from build123d import *

# Parameters (mm, degrees)
EXTRUDE_1_DEPTH     = 20
SKETCH_2_R          = 1.5
CUT_EXTRUDE_1_DEPTH = 20
SKETCH_3_R          = 7.5
EXTRUDE_2_DEPTH     = 50
EXTRUDE_3_DEPTH     = 10
SKETCH_7_W          = 18
SKETCH_7_H          = 39
EXTRUDE_4_DEPTH     = 5
SKETCH_9_R          = 5
SKETCH_9_R_2        = 1.75
CUT_EXTRUDE_2_DEPTH = 15
SKETCH_12_R         = 4
CUT_EXTRUDE_3_DEPTH = 20
CUT_EXTRUDE_START   = -60.849857
SKETCH_13_W         = 10
SKETCH_13_H         = 24
CUT_EXTRUDE_4_DEPTH = 60.849857
SKETCH_14_R         = 1.75
CUT_EXTRUDE_5_DEPTH = 10


with BuildPart() as part:
    # 草图1 → 凸台-拉伸1 (new body)
    with BuildSketch(Plane.XY):
        Polygon((-18, 29.079835166), (-13.000041786, 24.079835166), (-13.000343311, -12.000164834), (-10.85, -12.000164834), (-8.85, -14.000164834), (11.15, -14.000164834), (13.15, -12.000164834), (19.15, -12.000164834), (21.15, -14.000164834), (21.15, -28.920164834), (-73.85, -28.920164834), (-73.85, 29.079835166), align=None)
    extrude(amount=EXTRUDE_1_DEPTH)

    # 草图2 → 切除-拉伸1 (cut)
    with BuildSketch(Plane.XY.offset(20)):
        with Locations((-15.5, 15.5)):
            Circle(SKETCH_2_R)
        with Locations((-15.5, -15.5)):
            Circle(SKETCH_2_R)
        with Locations((15.5, -15.5)):
            Circle(SKETCH_2_R)
    extrude(amount=-CUT_EXTRUDE_1_DEPTH, mode=Mode.SUBTRACT)

    # 草图3 → 凸台-拉伸2 (add)
    with BuildSketch(Plane.XZ.offset(28.920164834)):
        with BuildLine():
            Line((-43.15, 31), (-43.15, 20))
            Line((-43.15, 20), (-21.15, 20))
            Line((-21.15, 20), (-21.15, 31))
            ThreePointArc((-21.15, 31), (-32.15, 42), (-43.15, 31))
        make_face()
        with Locations((-32.15, 31)):
            Circle(SKETCH_3_R, mode=Mode.SUBTRACT)
    extrude(amount=-EXTRUDE_2_DEPTH)

    # 草图5 → 凸台-拉伸3 (add)
    with BuildSketch(Plane.XZ.offset(28.920164834)):
        with BuildLine():
            Line((-43.15, 42), (-32.15, 42))
            ThreePointArc((-32.15, 42), (-39.928174593, 38.778174593), (-43.15, 31))
            Line((-43.15, 31), (-43.15, 20))
            Line((-43.15, 20), (-65.15, 20))
            Line((-65.15, 20), (-65.15, 37))
            ThreePointArc((-65.15, 37), (-63.685533906, 40.535533906), (-60.15, 42))
            Line((-60.15, 42), (-43.15, 42))
        make_face()
    extrude(amount=-EXTRUDE_3_DEPTH)

    # 草图7 → 凸台-拉伸4 (add)
    with BuildSketch(Plane.XY.offset(20)):
        with Locations((-82.85, -9.420164834)):
            Rectangle(SKETCH_7_W, SKETCH_7_H)
    extrude(amount=-EXTRUDE_4_DEPTH)

    # 草图9 → 切除-拉伸2 (cut)
    with BuildSketch(Plane.XZ.offset(28.920164834)):
        with Locations((-54.15, 31)):
            Circle(SKETCH_9_R)
        with Locations((-59.806854249, 36.656854249)):
            Circle(SKETCH_9_R_2)
        with Locations((-48.493145751, 36.656854249)):
            Circle(SKETCH_9_R_2)
        with Locations((-48.493145751, 25.343145751)):
            Circle(SKETCH_9_R_2)
        with Locations((-59.806854249, 25.343145751)):
            Circle(SKETCH_9_R_2)
    extrude(amount=-CUT_EXTRUDE_2_DEPTH, mode=Mode.SUBTRACT)

    # 草图12 → 切除-拉伸3 (cut)
    with BuildSketch(Plane.ZY.offset(73.85)):
        with Locations((10, 22.579835166)):
            Circle(SKETCH_12_R)
        with Locations((10, -22.420164834)):
            Circle(SKETCH_12_R)
    extrude(amount=-CUT_EXTRUDE_3_DEPTH, mode=Mode.SUBTRACT)

    # 草图13 → 切除-拉伸4 (cut)
    with BuildSketch(Plane.ZY.offset(73.85).offset(CUT_EXTRUDE_START)):
        with Locations((10, 0)):
            Rectangle(SKETCH_13_W, SKETCH_13_H)
    extrude(amount=CUT_EXTRUDE_4_DEPTH, mode=Mode.SUBTRACT)

    # 草图14 → 切除-拉伸5 (cut)
    with BuildSketch(Plane.XY.offset(20)):
        with Locations((-88.6, -12.170164834)):
            Circle(SKETCH_14_R)
        with Locations((-88.6, 6.829835166)):
            Circle(SKETCH_14_R)
    extrude(amount=-CUT_EXTRUDE_5_DEPTH, mode=Mode.SUBTRACT)


solid = part.part
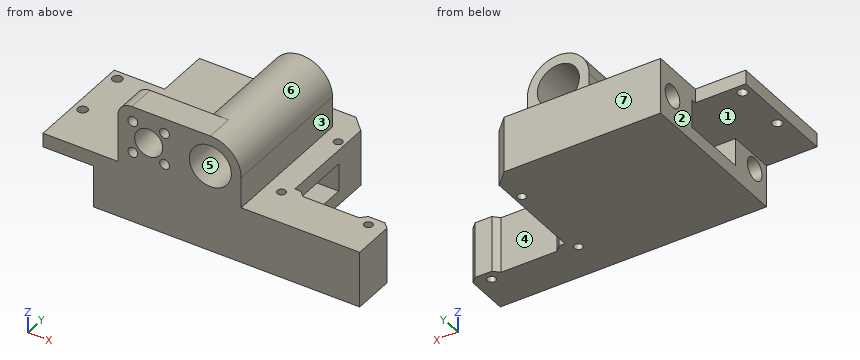
Part model, mm, in its own coordinate system. Face numbers are marked on the shaded views. A direction names the side the tool comes from. Coordinates: 2 decimals unless noted, no trailing zeros. Loops run counter-clockwise (first coordinate to the right, second up) from the corner with the lowest first, then second, coordinate; pieces in that order, holes last. Notation, with made-up numbers: (21.5, 71) -> (48.5, 71) arc R20 cw to (48.5, 78) -> close; hole circle Ø2 at (43, -16). An arc over 180 degrees is marked (long way). Use a Markdown table: item, result. Add a question column.
Item 1: Which spindle directions (+Z, -Z, +X, -X, +Y, -Y) get a long thin tool onto all of the face, cutting with end or side? Do the marked faces 1, 2, 3 and 4. Say none if no direction does.
Item 2: Band-saw the part on C-C on x = -88.6. Write the cut outline in (y, z).
Item 3: Probe probe 1 along Y at (x, z) = (-15.5, 4.75); probe 2 along Z at (x, y) = (-32.15, 0.5); probe 3 along Y at (x, z) = (-59, 10). List the from-to ranges inside material, lowest first.
Item 4: Band-saw the part on A-A on z = 10. Give the number of separate pieces and of enclosed holes in the cut face, plus the area to 3 significant figures.
Item 5: Band-saw the part on B-B on y = 15.5. Write the cut outline in (x, z), plus the area to 3 significant figures.
Item 6: Band-saw the part on D-D on z = 3. Write the cut outline in (x, y), plus the area to 3 significant figures.
Item 7: Flat gauge pins, fed straight in: P1, Ø17.5, axis at x = -29, z = 29.5, coming from the +Y side; P2, Ø3, axis at x = -76.5, y = 22.5, coming from the +Z side; P3, Ø3, axis at x = 15, z = 14, coming from the +Y side; P4, Ø9, axis at y = 22.5, z = 9.5, coming from the -X side. Where does each tip first touch, or does it go through?
Item 8: Pull direction X, two halves, no side cores. Call the marked faces 5, 6 and 7: +X half, -X half, draft (parallel to the pull), parting line (faces both ways), or undercut.
Geometry says:
| question | item | result |
|---|---|---|
| 1 | face 1 | -X |
| 1 | face 2 | -Z, -X, +Y |
| 1 | face 3 | +Z, +X, +Y, -Y |
| 1 | face 4 | +Z, -Z, +Y |
| 2 | outline | (-28.92, 15) -> (-13.92, 15) -> (-13.92, 20) -> (-28.92, 20) -> close; (-10.42, 15) -> (5.08, 15) -> (5.08, 20) -> (-10.42, 20) -> close; (8.58, 15) -> (10.08, 15) -> (10.08, 20) -> (8.58, 20) -> close |
| 3 | probe 1 | -28.92 to -17, -14 to 14, 17 to 26.58 |
| 3 | probe 2 | 0 to 5, 15 to 23.5, 38.5 to 42 |
| 3 | probe 3 | -28.92 to -26.42, -18.42 to -12, 12 to 18.58, 26.58 to 29.08 |
| 4 | separate pieces | 2 |
| 4 | enclosed holes | 3 |
| 4 | area | 2,250 mm² |
| 5 | outline | (-73.85, 0) -> (-17, 0) -> (-17, 20) -> (-21.15, 20) -> (-21.15, 31) arc R11 ccw to (-43.15, 31) -> (-43.15, 20) -> (-73.85, 20) -> close; (-14, 0) -> (-13, 0) -> (-13, 20) -> (-14, 20) -> close; hole circle Ø15 at (-32.15, 31) |
| 5 | area | 1,410 mm² |
| 6 | outline | (-73.85, -28.92) -> (21.15, -28.92) -> (21.15, -14) -> (19.15, -12) -> (13.15, -12) -> (11.15, -14) -> (-8.85, -14) -> (-10.85, -12) -> (-13, -12) -> (-13, 24.08) -> (-18, 29.08) -> (-73.85, 29.08) -> close; hole circle Ø3 at (-15.5, -15.5); hole circle Ø3 at (-15.5, 15.5); hole circle Ø3 at (15.5, -15.5) |
| 6 | area | 4,030 mm² |
| 7 | P1 | y = 21.08 |
| 7 | P2 | through |
| 7 | P3 | y = -12 |
| 7 | P4 | x = -73.85 |
| 8 | face 5 | undercut |
| 8 | face 6 | parting line |
| 8 | face 7 | draft |
